Part model, mm, in its own coordinate system. A direction names the side the tool comes from. Round coordinates to 2 decimals unless told otherwise and drop trailing zeros. Write each loop counter-clockwise with the first axis right and the second up, starting at its lowest first coordinate (ties: lowest second). Pieces come first, ordered by that corner, then holes.
1) Saw through at B-B on z = -1.5. Write the cut outline in (x, y) (3 decimals), and give its area (3 significant figures).
2) Saw through at D-D on x = 3.5. Write the cut outline in (y, z) (3 decimals).
3) Drill centre lines: L1, parallel to Y at x = -3, z = -5.75 (3 decimals); L2, parallel to Z at x = 3.5, y = 0.25; L3, parallel to X at y = -0.5, z = -0.5. Where is each one in solid material? Low to high.
4) Saw through at A-A on x = 5. Write the cut outline in (y, z) (3 decimals), and give its area (3 significant figures).
5) Saw through at C-C on x = -4.25. Write the cut outline in (y, z) (3 decimals).
6) Which spindle directions (+Z, -Z, +X, -X, +Y, -Y) get a long thin tool onto all of the face, cutting with end or side? Do faces 1 (the flat face through (0, 0, 5.81)), 2 (the flat face through (0, -0.6, -5)). Say none if no direction does.
```python
from build123d import *

# Parameters (mm, degrees)
SKETCH2_W           = 14.5
SKETCH2_H           = 11.62
BOSS_EXTRUDE1_DEPTH = 0.425
SKETCH6_W           = 13.5
SKETCH6_H           = 8.1
BOSS_EXTRUDE2_DEPTH = 0.2
SKETCH7_W           = 12.58
SKETCH7_H           = 6.98
BOSS_EXTRUDE3_DEPTH = 0.15
BOSS_EXTRUDE4_DEPTH = 0.17547
FILLET1_R           = 0.762
FILLET2_R           = 0.2
SKETCH13_W          = 8
SKETCH13_H          = 0.1
BOSS_EXTRUDE5_DEPTH = 10
SKETCH20_W          = 1.79
SKETCH20_H          = 5
SKETCH20_W_2        = 2.21
BOSS_EXTRUDE6_DEPTH = 0.1
SKETCH23_R          = 0.5
CUT_EXTRUDE1_DEPTH  = 0.1
FILLET3_R           = 1
FILLET4_R           = 0.5
FILLET5_R           = 0.5


with BuildPart() as part:
    # Sketch2 → Boss-Extrude1 (new, symmetric)
    with BuildSketch(Plane(origin=(0, 0, 0), x_dir=(1, 0, 0), z_dir=(0, 1, 0))):
        Rectangle(SKETCH2_W, SKETCH2_H)
    extrude(amount=BOSS_EXTRUDE1_DEPTH, both=True)

    # Sketch6 → Boss-Extrude2 (add)
    with BuildSketch(Plane.XZ.offset(0.425)):
        with Locations((0, 1.76)):
            Rectangle(SKETCH6_W, SKETCH6_H)
    extrude(amount=BOSS_EXTRUDE2_DEPTH)

    # Sketch7 → Boss-Extrude3 (add)
    with BuildSketch(Plane.XZ.offset(0.625)):
        with Locations((0, 1.51)):
            Rectangle(SKETCH7_W, SKETCH7_H)
    extrude(amount=BOSS_EXTRUDE3_DEPTH)

    # Sketch9 → Boss-Extrude4 (add)
    with BuildSketch(Plane.XZ.offset(0.425)):
        Polygon((-6.096, -2.452696), (6.096, -2.452696), (6.096, -4.992696), (3.2893, -4.992696), (3.2893, -7.856286), (-3.2893, -7.856286), (-3.2893, -4.992696), (-6.096, -4.992696), align=None)
    extrude(amount=BOSS_EXTRUDE4_DEPTH)

    # Fillet1
    fillet1_edges = [part.edges().sort_by_distance(p)[0] for p in [
        (6.096, -0.512735, -4.992696),
        (-6.096, -0.512735, -4.992696),
    ]]
    fillet(fillet1_edges, radius=FILLET1_R)

    # Fillet2
    fillet2_edges = [part.edges().sort_by_distance(p)[0] for p in [
        (-3.2893, -0.512735, -7.856286),
        (3.2893, -0.512735, -7.856286),
    ]]
    fillet(fillet2_edges, radius=FILLET2_R)

    # Sketch13 → Boss-Extrude5 (add)
    with BuildSketch(Plane(origin=(0, 0, -5.81), x_dir=(-1, 0, 0), z_dir=(0, 0, -1))):
        with Locations((0, -0.375)):
            Rectangle(SKETCH13_W, SKETCH13_H)
    extrude(amount=BOSS_EXTRUDE5_DEPTH)

    # Sketch20 → Boss-Extrude6 (add)
    with BuildSketch(Plane.XZ.offset(0.425)):
        with Locations((-4.895, -13.31)):
            Rectangle(SKETCH20_W, SKETCH20_H)
        with Locations((5.105, -13.31)):
            Rectangle(SKETCH20_W_2, SKETCH20_H)
    extrude(amount=-BOSS_EXTRUDE6_DEPTH)

    # Sketch23 → Cut-Extrude1 (cut)
    with BuildSketch(Plane(origin=(0, -0.325, 0), x_dir=(1, 0, 0), z_dir=(0, 1, 0))):
        with Locations(Location((5, 11.81, 0), (0, 0, 270))):
            Circle(SKETCH23_R)
        with Locations(Location((-5, 11.81, 0), (0, 0, 270))):
            Circle(SKETCH23_R)
    extrude(amount=-CUT_EXTRUDE1_DEPTH, mode=Mode.SUBTRACT)

    # Fillet3
    fillet3_edges = [part.edges().sort_by_distance(p)[0] for p in [
        (-5.79, -0.375, -10.81),
        (6.21, -0.375, -10.81),
    ]]
    fillet(fillet3_edges, radius=FILLET3_R)

    # Fillet4
    fillet4_edges = [part.edges().sort_by_distance(p)[0] for p in [
        (-5.79, -0.375, -15.81),
        (6.21, -0.375, -15.81),
    ]]
    fillet(fillet4_edges, radius=FILLET4_R)

    # Fillet5
    fillet5_edges = [part.edges().sort_by_distance(p)[0] for p in [
        (-4, -0.375, -10.81),
        (4, -0.375, -10.81),
    ]]
    fillet(fillet5_edges, radius=FILLET5_R)


solid = part.part
```
Completed:
1. outline: (-7.25, -0.425) - (-6.75, -0.425) - (-6.75, -0.625) - (-6.29, -0.625) - (-6.29, -0.775) - (6.29, -0.775) - (6.29, -0.625) - (6.75, -0.625) - (6.75, -0.425) - (7.25, -0.425) - (7.25, 0.425) - (-7.25, 0.425) - close
1. area: 16.9 mm2
2. outline: (-0.775, -1.98) - (-0.625, -1.98) - (-0.625, -2.29) - (-0.425, -2.29) - (-0.425, -2.453) - (-0.6, -2.453) - (-0.6, -4.993) - (-0.425, -4.993) - (-0.425, -15.81) - (-0.325, -15.81) - (-0.325, -5.81) - (0.425, -5.81) - (0.425, 5.81) - (-0.625, 5.81) - (-0.625, 5) - (-0.775, 5) - close
3. L1: y = -0.6 to 0.425
3. L2: z = -5.81 to 5.81
3. L3: x = -6.75 to 6.75
4. outline: (-0.775, -1.98) - (-0.625, -1.98) - (-0.625, -2.29) - (-0.425, -2.29) - (-0.425, -2.453) - (-0.6, -2.453) - (-0.6, -4.993) - (-0.425, -4.993) - (-0.425, -5.81) - (0.425, -5.81) - (0.425, 5.81) - (-0.625, 5.81) - (-0.625, 5) - (-0.775, 5) - close; (-0.425, -15.81) - (-0.325, -15.81) - (-0.325, -12.31) - (-0.425, -12.31) - close; (-0.425, -11.31) - (-0.325, -11.31) - (-0.325, -10.81) - (-0.425, -10.81) - close
4. area: 13.4 mm2
5. outline: (-0.775, -1.98) - (-0.625, -1.98) - (-0.625, -2.29) - (-0.425, -2.29) - (-0.425, -2.453) - (-0.6, -2.453) - (-0.6, -4.993) - (-0.425, -4.993) - (-0.425, -5.81) - (0.425, -5.81) - (0.425, 5.81) - (-0.625, 5.81) - (-0.625, 5) - (-0.775, 5) - close; (-0.425, -15.81) - (-0.325, -15.81) - (-0.325, -10.743) - (-0.425, -10.743) - close
6. face 1: +Z, +X, -X, +Y, -Y
6. face 2: -Z, +X, -X, -Y
